```python
from build123d import *

# Parameters (mm, degrees)
BOSS_EXTRU_1_START = -2
BOSS_EXTRU_1_DEPTH = 2
CONG_1_R           = 1
CONG_3_R           = 0.5


with BuildPart() as part:
    # Esquisse1 → Révolution1 (revolve)
    with BuildSketch(Plane.XY, mode=Mode.PRIVATE) as r_volution1_sk:
        Polygon((0, 4.05), (0, 5.95), (2, 5.95), (2, 4.95), (5, 4.95), (5, 4.05), align=None)
    revolve(r_volution1_sk.sketch.rotate(Axis((-3.996004355, 0, 0), (1, 0, 0)), 90), axis=Axis((-3.996004355, 0, 0), (1, 0, 0)))

    # Esquisse2 → Boss.-Extru.1 (add)
    with BuildSketch(Plane.ZY.offset(BOSS_EXTRU_1_START)):
        with BuildLine():
            Line((5.85960613, -1.033206657), (9.798837142, -1.727799368))
            ThreePointArc((9.798837142, -1.727799368), (9.95, 0), (9.798837142, 1.727799368))
            Line((9.798837142, 1.727799368), (5.85960613, 1.033206657))
            ThreePointArc((5.85960613, 1.033206657), (5.95, 0), (5.85960613, -1.033206657))
        make_face()
    extrude(amount=BOSS_EXTRU_1_DEPTH)

    # Congé1
    cong_1_edges = [part.edges().sort_by_distance(p)[0] for p in [
        (1, -1.033206657, 5.85960613),
        (1, 1.033206657, 5.85960613),
    ]]
    fillet(cong_1_edges, radius=CONG_1_R)

    # Congé3
    cong_3_edges = [part.edges().sort_by_distance(p)[0] for p in [
        (1, 1.727799368, 9.798837142),
        (1, -1.727799368, 9.798837142),
    ]]
    fillet(cong_3_edges, radius=CONG_3_R)


solid = part.part
```
Read the model definition and answer for the solid it produces. Units are mm, in the model's axes. A direction names the side the tool comes from. Give positions to 0.01 mm unless a question says otherwise; leave off trailing zeros. Write each loop counter-clockwise with the first axis right and the second up, starting at its lowest first coordinate (ties: lowest second). Pieces come first, ordered by that corner, then holes. Notation, with made-up numbers: (4.5, -30) -> (23.5, -30) arc R17 cw to (23.5, -18) -> close; hole circle Ø7 at (17, -3.75). An arc over 180 degrees is marked (long way). Answer as a JSON object with one key per item and string values.
1) Section C-C on x = 1.2 is taken. Write down the section's boundary in (y, z).
Findings below:
{"outline": "(-1.87, 5.65) arc R5.95 ccw (long way) to (1.87, 5.65) arc R1 cw to (1.19, 6.77) -> (1.64, 9.29) arc R0.5 ccw to (1.21, 9.88) arc R9.95 ccw to (-1.21, 9.88) arc R0.5 ccw to (-1.64, 9.29) -> (-1.19, 6.77) arc R1 cw to start; hole circle Ø8.1 at (0, 0)"}
2) Section A-A on z = 0 is taken. Write down the section's boundary in (x, y), then the cut area to 3 significant figures.
Findings below:
{"outline": "(0, -5.95) -> (2, -5.95) -> (2, -4.95) -> (5, -4.95) -> (5, -4.05) -> (0, -4.05) -> close; (0, 4.05) -> (5, 4.05) -> (5, 4.95) -> (2, 4.95) -> (2, 5.95) -> (0, 5.95) -> close", "area": "13.0 mm^2"}
3) A tool of negligible diameter and unlimited length cuts with its end or side. For faces 4 (the flat face through (5, 4, -2)), 5 (the flat face through (1.01, 1.42, 8.05)), 6 (the flat face through (2, 2, 5)), 7 (the flat face through (1.014, -1.413, 8.016)), from which of +Z, -Z, +X, -X, +Y, -Y can it reach the whole face along a straight path? Write none if from no direction.
Findings below:
{"face 4": "+Z, -Z, +X, +Y, -Y", "face 5": "+X, -X, +Y", "face 6": "+X", "face 7": "+X, -X, -Y"}
4) Flat-ended cylindrical pins translate along their axes: pin 1 Ø1.5 at (x, y) = (4, 0.5) entering from -Z; pin 2 Ø2 at (x, z) = (2, -4) entering from -Y. Find the tip coordinate at first contact, or state that the pin passes through.
Findings below:
{"pin 1": "stops at z = -4.95", "pin 2": "stops at y = -5.14"}
5) Straight lines are drawn through the part: probe 1 along Y at (x, z) = (2.55, 0); probe 2 along X at (y, z) = (-4.5, 3.5); probe 3 along Z at (x, y) = (2.2, 2.75). For each, find the intervals that lie inside material, in ascending order. Write a range as from..to.
Findings below:
{"probe 1": "y = -4.95..-4.05, 4.05..4.95", "probe 2": "x = 0..2", "probe 3": "z = -4.12..-2.97, 2.97..4.12"}
6) Section D-D on x = 2.95 is taken. Write down the section's boundary in (y, z), then the cut area to 3 significant figures.
Findings below:
{"outline": "circle Ø9.9 at (0, 0); hole circle Ø8.1 at (0, 0)", "area": "25.4 mm^2"}
7) Section B-B on y = 0 is taken. Write down the section's boundary in (x, z), then the cut area to 3 significant figures.
Findings below:
{"outline": "(0, -5.95) -> (2, -5.95) -> (2, -4.95) -> (5, -4.95) -> (5, -4.05) -> (0, -4.05) -> close; (0, 4.05) -> (5, 4.05) -> (5, 4.95) -> (2, 4.95) -> (2, 9.95) -> (0, 9.95) -> close", "area": "21.0 mm^2"}
8) For a pull along Z with two mould halves and no side action, classify faces 1 (the flat face through (0, 3, 4)), 2 (the cylindrical face through (3.52, -1.49, 4.72)), 3 (the cylindrical face through (0.986, 1.326, 6.078)) as pulls with the +Z half, pulls with the -Z half, needs draft (parallel to the pull), parting line crosses it, or undercut.
Findings below:
{"face 1": "needs draft", "face 2": "parting line crosses it", "face 3": "undercut"}
